```python
from build123d import *

# Parameters (mm, degrees)
CROQUIS1_R              = 4
SALIENTE_EXTRUIR1_DEPTH = 1.5
CROQUIS2_R              = 5
CROQUIS2_R_2            = 1
CROQUIS2_W              = 6
CROQUIS2_H              = 11
CORTAR_EXTRUIR1_DEPTH   = 3
CROQUIS3_R              = 1.5875
CROQUIS3_R_2            = 1.590536349
CORTAR_EXTRUIR2_DEPTH   = 23


with BuildPart() as part:
    # Croquis1 → Saliente-Extruir1 (new, symmetric)
    with BuildSketch(Plane(origin=(0, 0, 0), x_dir=(1, 0, 0), z_dir=(0, 1, 0))):
        Polygon((-77, -42), (-77, -54), (77, -54), (77, -42), (74, -42), (74, -28), (77, -28), (77, -20), (74, -20), (74, -12), (77, -12), (77, -4), (74, -4), (74, -1.5), (74, 1.5), (74, 4), (77, 4), (77, 12), (74, 12), (74, 14.5), (70.25, 14.5), (70.25, 12), (67.25, 12), (67.25, 14.5), (66.27, 14.5), (66.27, 17.5), (67.25, 17.5), (67.25, 20), (70.25, 20), (70.25, 17.5), (74, 17.5), (74, 20), (77, 20), (77, 28), (74, 28), (74, 42), (77, 42), (77, 54), (65, 54), (65, 51), (55, 51), (55, 54), (45, 54), (45, 51), (31.5, 51), (31.5, 47.25), (34, 47.25), (34, 44.25), (31.5, 44.25), (31.5, 43.27), (28.5, 43.27), (28.5, 44.25), (26, 44.25), (26, 47.25), (28.5, 47.25), (28.5, 51), (15, 51), (15, 54), (5, 54), (5, 51), (-5, 51), (-5, 54), (-15, 54), (-15, 51), (-28.5, 51), (-28.5, 47.25), (-26, 47.25), (-26, 44.25), (-28.5, 44.25), (-28.5, 43.27), (-31.5, 43.27), (-31.5, 44.25), (-34, 44.25), (-34, 47.25), (-31.5, 47.25), (-31.5, 51), (-45, 51), (-45, 54), (-55, 54), (-55, 51), (-65, 51), (-65, 54), (-77, 54), (-77, 42), (-74, 42), (-74, 28), (-77, 28), (-77, 20), (-74, 20), (-74, 17.5), (-70.25, 17.5), (-70.25, 20), (-67.25, 20), (-67.25, 17.5), (-66.27, 17.5), (-66.27, 14.5), (-67.25, 14.5), (-67.25, 12), (-70.25, 12), (-70.25, 14.5), (-74, 14.5), (-74, 12), (-77, 12), (-77, 4), (-74, 4), (-74, 1.5), (-74, -1.5), (-74, -4), (-77, -4), (-77, -12), (-74, -12), (-74, -20), (-77, -20), (-77, -28), (-74, -28), (-74, -42), align=None)
        with Locations(Location((-65, -48, 0), (0, 0, 270))):
            Circle(CROQUIS1_R, mode=Mode.SUBTRACT)
        with BuildLine():
            Line((55, -49.6), (53, -49.6))
            ThreePointArc((53, -49.6), (52.646446609, -49.453553391), (52.5, -49.1))
            Line((52.5, -49.1), (52.5, -46.4))
            Line((52.5, -46.4), (55.5, -46.4))
            Line((55.5, -46.4), (55.5, -49.1))
            ThreePointArc((55.5, -49.1), (55.353553391, -49.453553391), (55, -49.6))
        make_face(mode=Mode.SUBTRACT)
    extrude(amount=SALIENTE_EXTRUIR1_DEPTH, both=True)

    # Croquis2 → Cortar-Extruir1 (cut)
    with BuildSketch(Plane(origin=(0, 1.5, 0), x_dir=(1, 0, 0), z_dir=(0, 1, 0))):
        with Locations(Location((-5, -32.83, 0), (0, 0, 270))):
            Circle(CROQUIS2_R)
        with Locations(Location((10.51, 37.3, 0), (0, 0, 270))):
            Circle(CROQUIS2_R_2)
        with Locations(Location((52.51, 37.3, 0), (0, 0, 270))):
            Circle(CROQUIS2_R_2)
        with Locations(Location((52.51, -34.7, 0), (0, 0, 270))):
            Circle(CROQUIS2_R_2)
        with Locations(Location((10.51, -34.7, 0), (0, 0, 270))):
            Circle(CROQUIS2_R_2)
        with Locations((-34.16, 4.52)):
            Rectangle(CROQUIS2_W, CROQUIS2_H)
        with Locations((-5, 33.81)):
            Rectangle(CROQUIS2_W, CROQUIS2_H)
        with Locations((-44.16, 4.52)):
            Rectangle(CROQUIS2_W, CROQUIS2_H)
        with Locations((-44.16, 19.52)):
            Rectangle(CROQUIS2_W, CROQUIS2_H)
        with Locations((-34.16, 19.52)):
            Rectangle(CROQUIS2_W, CROQUIS2_H)
        with Locations((-5, 11.63)):
            Rectangle(CROQUIS2_W, CROQUIS2_H)
        with Locations((-5, -10.55)):
            Rectangle(CROQUIS2_W, CROQUIS2_H)
        with Locations((21.51, 18.3)):
            Rectangle(CROQUIS2_W, CROQUIS2_H)
        with Locations((41.51, 18.3)):
            Rectangle(CROQUIS2_W, CROQUIS2_H)
        with Locations((41.51, -11.7)):
            Rectangle(CROQUIS2_W, CROQUIS2_H)
        with Locations((21.51, -11.7)):
            Rectangle(CROQUIS2_W, CROQUIS2_H)
        with Locations((65, 39.36)):
            Rectangle(CROQUIS2_W, CROQUIS2_H)
        with Locations((65, -11.64)):
            Rectangle(CROQUIS2_W, CROQUIS2_H)
        with Locations((65, -39.64)):
            Rectangle(CROQUIS2_W, CROQUIS2_H)
        with Locations((65, 3.36)):
            Rectangle(CROQUIS2_W, CROQUIS2_H)
        with Locations((-65, 3.36)):
            Rectangle(CROQUIS2_W, CROQUIS2_H)
        with Locations((-65, 39.36)):
            Rectangle(CROQUIS2_W, CROQUIS2_H)
    extrude(amount=-CORTAR_EXTRUIR1_DEPTH, mode=Mode.SUBTRACT)

    # Croquis3 → Cortar-Extruir2 (cut)
    with BuildSketch(Plane(origin=(0, 1.5, 0), x_dir=(1, 0, 0), z_dir=(0, 1, 0))):
        with Locations(Location((-60.888852319, -11.348115731, 0), (0, 0, 270))):
            Circle(CROQUIS3_R)
        with Locations(Location((-12.628852319, -12.618115731, 0), (0, 0, 270))):
            Circle(CROQUIS3_R)
        with Locations(Location((-45.648852319, 39.451884269, 0), (0, 0, 270))):
            Circle(CROQUIS3_R)
        with Locations(Location((-17.708852319, 39.451884269, 0), (0, 0, 270))):
            Circle(CROQUIS3_R_2)
    extrude(amount=-CORTAR_EXTRUIR2_DEPTH, mode=Mode.SUBTRACT)


solid = part.part
```
Work out the finished part from the listing and answer in its coordinate system (mm). A direction names the side the tool comes from. Round coordinates to 2 decimals unless told otherwise and drop trailing zeros. Return JSON: item names as keys, results as strings. Group by question number.
Q1. The part is cut by section A-A on y = 0.95. Count the separate pieces of the cut face and the enclosed holes in it, then the cut area to 3 significant figures.
Q2. Find the intervals of material crossed by L1, parallel to X at y = -0.95, z = -12.5; L2, parallel to X at y = 0, z = -45; L3, parallel to X at y = 0.55, z = -37.3, in increasing order.
Q3. For faces 1 (the flat face through (77, 0, 24)), 2 (the flat face through (75, 0, -4)), 3 (the flat face through (-68, 0, -3)), 4 (the flat face through (-75, 0, -12)), determine the directions among +Z, -Z, +X, -X, +Y, -Y from which every point of the face is accessible in a straight line to the end or side of a thin tool.
Q4. The mould has two halves that part along X. Classify faces 5 (the flat face through (77, 0, -24)), 6 (the flat face through (-1, 0, 54)), 7 (the flat face through (41, 0, -12.8)), 8 (the flat face through (-65, 0, 2.14)): released by +X, released by -X, zero draft, split by the parting line, or undercut.
Q5. Each of these flat-tipped pins is pushed along its axis until it touches: pin 1 Ø1 at (y, z) = (0.5, 16.5) entering from +X; pin 2 Ø1 at (y, z) = (0, -1.5) entering from -X; pin 3 Ø1.2 at (x, z) = (10.51, -37.3) entering from -Y. Where does it stop, or does it pass through?
Solved:
{
 "1": {"separate pieces": "1", "enclosed holes": "28", "area": "14,600 mm²"},
 "2": {"L1": "-74 to -70.25, -67.25 to -8, -2 to 67.25, 70.25 to 74", "L2": "-77 to -34, -26 to 26, 34 to 77", "L3": "-74 to -68, -62 to -8, -2 to 9.51, 11.51 to 51.51, 53.51 to 62, 68 to 74"},
 "3": {"face 1": "+Z, -Z, +X, +Y, -Y", "face 2": "+X, +Y, -Y", "face 3": "+Y, -Y", "face 4": "-X, +Y, -Y"},
 "4": {"face 5": "released by +X", "face 6": "zero draft", "face 7": "undercut", "face 8": "undercut"},
 "5": {"pin 1": "x = 74", "pin 2": "x = -74", "pin 3": "through"}
}
